```python
from build123d import *

# Parameters (mm, degrees)
DODANIE_WYCI_GNI_CIE1_DEPTH = 10
WYTNIJ_WYCI_GNI_CIE1_DEPTH  = 10


with BuildPart() as part:
    # Szkic1 → Dodanie-wyciągnięcie1 (new body)
    with BuildSketch(Plane.XY):
        with BuildLine():
            Line((-39.146316842, 3.9), (-57.146316842, 3.9))
            Line((-57.146316842, 3.9), (-57.146316842, 26.7))
            ThreePointArc((-57.146316842, 26.7), (-56.560530404, 28.114213562), (-55.146316842, 28.7))
            Line((-55.146316842, 28.7), (-47.146316842, 28.7))
            Line((-47.146316842, 28.7), (-47.146316842, 39.1))
            Line((-47.146316842, 39.1), (-55.146316842, 39.1))
            ThreePointArc((-55.146316842, 39.1), (-56.560530404, 39.685786438), (-57.146316842, 41.1))
            Line((-57.146316842, 41.1), (-57.146316842, 47))
            Line((-57.146316842, 47), (-39.146316842, 47))
            Line((-39.146316842, 47), (-39.146316842, 3.9))
        make_face()
    extrude(amount=DODANIE_WYCI_GNI_CIE1_DEPTH)

    # Szkic2 → Wytnij-wyciągnięcie1 (cut)
    with BuildSketch(Plane.XY.offset(10)):
        Polygon((-46.596316842, 3.9), (-46.596316842, 7.6), (-45.221316842, 7.6), (-45.221316842, 9.6), (-46.596316842, 9.6), (-46.596316842, 10.1), (-49.696316842, 10.1), (-49.696316842, 9.6), (-51.071316842, 9.6), (-51.071316842, 7.6), (-49.696316842, 7.6), (-49.696316842, 3.9), align=None)
    extrude(amount=-WYTNIJ_WYCI_GNI_CIE1_DEPTH, mode=Mode.SUBTRACT)


solid = part.part
```
Work out the finished part from the listing and answer in its coordinate system (mm). A direction names the side the tool comes from. Coordinates: 2 decimals unless noted, no trailing zeros. Write each loop counter-clockwise with the first axis right and the second up, starting at its lowest first coordinate (ties: lowest second). Pieces come first, ordered by that corner, then holes.
Q1. Each of these flat-tipped pins is pushed along its axis until it touches: pin 1 Ø2 at (y, z) = (32.5, 7) entering from -X; pin 2 Ø3 at (y, z) = (39.5, 7.5) entering from -X. Where does it stop, or does it pass through?
Q2. A cutting plane is placed at B-B, the plane z = 3.25. Give the vertices of the cut face in (x, y), then the cut area to 3 significant figures.
Q3. A cutting plane is placed at C-C, the plane y = 31.5. Give the vertices of the cut face in (x, z), then the cut area to 3 significant figures.
Q4. Find the intervals of material crossed by line 1 (Y direction, x = -52, z = 8.5); line 2 (Y direction, x = -51, z = 1.5); line 3 (Y direction, x = -48.5, z = 6.5), in increasing order.
Q5. Which of the six approach directions +Z, -Z, +X, -X, +Y, -Y give full straight-line access (tool end or side, diameter ignored) to faces 4 (the face through (-47.146, 34, 5)), 5 (the face through (-46.596, 6, 5)), 6 (the face through (-43, 3.9, 5)), 7 (the face through (-51.071, 9, 5)), 8 (the face through (-57.146, 44, 5))?
Q6. A cutting plane is placed at A-A, the plane x = -52.25. Give the vertices of the cut face in (y, z).
Q7. A cutting plane is placed at D-D, the plane x = -56. Give the vertices of the cut face in (y, z), then the cut area to 3 significant figures.
Q8. Determine the mould class of faces 1 (the face through (-48, 10.1, 5)), 2 (the face through (-50, 9.6, 5)), 3 (the face through (-49.696, 6, 5)) for opening direction Y: released by +Y, released by -Y, zero draft, split by the parting line, or undercut.
Findings below:
1. pin 1: stops at x = -47.15
1. pin 2: stops at x = -57.14
2. outline: (-57.15, 3.9) - (-49.7, 3.9) - (-49.7, 7.6) - (-51.07, 7.6) - (-51.07, 9.6) - (-49.7, 9.6) - (-49.7, 10.1) - (-46.6, 10.1) - (-46.6, 9.6) - (-45.22, 9.6) - (-45.22, 7.6) - (-46.6, 7.6) - (-46.6, 3.9) - (-39.15, 3.9) - (-39.15, 47) - (-57.15, 47) - (-57.15, 41.1) arc R2 ccw to (-55.15, 39.1) - (-47.15, 39.1) - (-47.15, 28.7) - (-55.15, 28.7) arc R2 ccw to (-57.15, 26.7) - close
2. area: 645 mm2
3. outline: (-47.15, 0) - (-39.15, 0) - (-39.15, 10) - (-47.15, 10) - close
3. area: 80.0 mm2
4. line 1: y = 3.9 to 28.7, 39.1 to 47
4. line 2: y = 3.9 to 7.6, 9.6 to 28.7, 39.1 to 47
4. line 3: y = 10.1 to 28.7, 39.1 to 47
5. face 4: +Z, -Z, -X
5. face 5: +Z, -Z, -Y
5. face 6: +Z, -Z, +X, -X, -Y
5. face 7: +Z, -Z
5. face 8: +Z, -Z, -X, +Y, -Y
6. outline: (3.9, 0) - (28.7, 0) - (28.7, 10) - (3.9, 10) - close; (39.1, 0) - (47, 0) - (47, 10) - (39.1, 10) - close
7. outline: (3.9, 0) - (28.51, 0) - (28.51, 10) - (3.9, 10) - close; (39.29, 0) - (47, 0) - (47, 10) - (39.29, 10) - close
7. area: 323 mm2
8. face 1: released by -Y
8. face 2: undercut
8. face 3: zero draft
